from build123d import *

# Parameters (mm, degrees)
SKETCH1_R           = 1.1
SKETCH1_R_2         = 1.55
BOSS_EXTRUDE1_DEPTH = 2
SKETCH2_R           = 1.55
SKETCH2_R_2         = 1.1
BOSS_EXTRUDE2_DEPTH = 2.5
BOSS_EXTRUDE3_START = -3
SKETCH3_W           = 15.5
SKETCH3_H           = 3.5
BOSS_EXTRUDE3_DEPTH = 3
SKETCH4_R           = 1.5
CUT_EXTRUDE1_DEPTH  = 5
CUT_EXTRUDE2_DEPTH  = 65.325422657
CUT_EXTRUDE3_DEPTH  = 106.250938238
CHAMFER1_SIZE       = 2.5


with BuildPart() as part:
    # Sketch1 → Boss-Extrude1 (new body)
    with BuildSketch(Plane(origin=(0, 0, 0), x_dir=(1, 0, 0), z_dir=(0, 1, 0))):
        with BuildLine():
            Line((-48, -42.4), (-43, -42.4))
            Line((-43, -42.4), (-35.267949192, -37.935898385))
            ThreePointArc((-35.267949192, -37.935898385), (-34.303225373, -37.536296695), (-33.267949192, -37.4))
            Line((-33.267949192, -37.4), (33.267949192, -37.4))
            ThreePointArc((33.267949192, -37.4), (34.303225373, -37.536296695), (35.267949192, -37.935898385))
            Line((35.267949192, -37.935898385), (43, -42.4))
            Line((43, -42.4), (48, -42.4))
            Line((48, -42.4), (48, 42.4))
            Line((48, 42.4), (43, 42.4))
            Line((43, 42.4), (35.267949192, 37.935898385))
            ThreePointArc((35.267949192, 37.935898385), (34.303225373, 37.536296695), (33.267949192, 37.4))
            Line((33.267949192, 37.4), (-33.267949192, 37.4))
            ThreePointArc((-33.267949192, 37.4), (-34.303225373, 37.536296695), (-35.267949192, 37.935898385))
            Line((-35.267949192, 37.935898385), (-43, 42.4))
            Line((-43, 42.4), (-48, 42.4))
            Line((-48, 42.4), (-48, -42.4))
        make_face()
        with Locations(Location((-13.5, -33.275, 0), (0, 0, 270))):
            Circle(SKETCH1_R, mode=Mode.SUBTRACT)
        with Locations(Location((-7.5, -33.275, 0), (0, 0, 270))):
            Circle(SKETCH1_R, mode=Mode.SUBTRACT)
        with Locations(Location((7.5, -33.275, 0), (0, 0, 270))):
            Circle(SKETCH1_R, mode=Mode.SUBTRACT)
        with Locations(Location((13.5, -33.275, 0), (0, 0, 270))):
            Circle(SKETCH1_R, mode=Mode.SUBTRACT)
        with Locations(Location((-13.5, 33.275, 0), (0, 0, 270))):
            Circle(SKETCH1_R, mode=Mode.SUBTRACT)
        with Locations(Location((-7.5, 33.275, 0), (0, 0, 270))):
            Circle(SKETCH1_R, mode=Mode.SUBTRACT)
        with Locations(Location((7.5, 33.275, 0), (0, 0, 270))):
            Circle(SKETCH1_R, mode=Mode.SUBTRACT)
        with Locations(Location((13.5, 33.275, 0), (0, 0, 270))):
            Circle(SKETCH1_R, mode=Mode.SUBTRACT)
        with Locations(Location((-42, 36.5, 0), (0, 0, 270))):
            Circle(SKETCH1_R_2, mode=Mode.SUBTRACT)
        with Locations(Location((42, 36.5, 0), (0, 0, 270))):
            Circle(SKETCH1_R_2, mode=Mode.SUBTRACT)
        with Locations(Location((42, -36.5, 0), (0, 0, 270))):
            Circle(SKETCH1_R_2, mode=Mode.SUBTRACT)
        with Locations(Location((-42, -36.5, 0), (0, 0, 270))):
            Circle(SKETCH1_R_2, mode=Mode.SUBTRACT)
        with BuildLine():
            Line((-37, 25.25), (-37, 9.75))
            ThreePointArc((-37, 9.75), (-41, 5.75), (-45, 9.75))
            Line((-45, 9.75), (-45, 25.25))
            ThreePointArc((-45, 25.25), (-41, 29.25), (-37, 25.25))
        make_face(mode=Mode.SUBTRACT)
        with BuildLine():
            Line((-37, -9.75), (-37, -25.25))
            ThreePointArc((-37, -25.25), (-41, -29.25), (-45, -25.25))
            Line((-45, -25.25), (-45, -9.75))
            ThreePointArc((-45, -9.75), (-41, -5.75), (-37, -9.75))
        make_face(mode=Mode.SUBTRACT)
        with BuildLine():
            Line((45, 25.25), (45, 9.75))
            ThreePointArc((45, 9.75), (41, 5.75), (37, 9.75))
            Line((37, 9.75), (37, 25.25))
            ThreePointArc((37, 25.25), (41, 29.25), (45, 25.25))
        make_face(mode=Mode.SUBTRACT)
        with BuildLine():
            Line((45, -9.75), (45, -25.25))
            ThreePointArc((45, -25.25), (41, -29.25), (37, -25.25))
            Line((37, -25.25), (37, -9.75))
            ThreePointArc((37, -9.75), (41, -5.75), (45, -9.75))
        make_face(mode=Mode.SUBTRACT)
    extrude(amount=BOSS_EXTRUDE1_DEPTH)

    # Sketch2 → Boss-Extrude2 (add)
    with BuildSketch(Plane(origin=(0, 2, 0), x_dir=(1, 0, 0), z_dir=(0, 1, 0))):
        with BuildLine():
            Line((48, -42.4), (48, 42.4))
            Line((48, 42.4), (43, 42.4))
            Line((43, 42.4), (35.267949192, 37.935898385))
            ThreePointArc((35.267949192, 37.935898385), (34.303225373, 37.536296695), (33.267949192, 37.4))
            Line((33.267949192, 37.4), (-33.267949192, 37.4))
            ThreePointArc((-33.267949192, 37.4), (-34.303225373, 37.536296695), (-35.267949192, 37.935898385))
            Line((-35.267949192, 37.935898385), (-43, 42.4))
            Line((-43, 42.4), (-48, 42.4))
            Line((-48, 42.4), (-48, -42.4))
            Line((-48, -42.4), (-43, -42.4))
            Line((-43, -42.4), (-35.267949192, -37.935898385))
            ThreePointArc((-35.267949192, -37.935898385), (-34.303225373, -37.536296695), (-33.267949192, -37.4))
            Line((-33.267949192, -37.4), (33.267949192, -37.4))
            ThreePointArc((33.267949192, -37.4), (34.303225373, -37.536296695), (35.267949192, -37.935898385))
            Line((35.267949192, -37.935898385), (43, -42.4))
            Line((43, -42.4), (48, -42.4))
        make_face()
        with Locations((-42, -36.5)):
            Circle(SKETCH2_R, mode=Mode.SUBTRACT)
        with Locations((-13.5, -33.275)):
            Circle(SKETCH2_R_2, mode=Mode.SUBTRACT)
        with Locations((-7.5, -33.275)):
            Circle(SKETCH2_R_2, mode=Mode.SUBTRACT)
        with Locations((7.5, -33.275)):
            Circle(SKETCH2_R_2, mode=Mode.SUBTRACT)
        with Locations((13.5, -33.275)):
            Circle(SKETCH2_R_2, mode=Mode.SUBTRACT)
        with Locations((42, -36.5)):
            Circle(SKETCH2_R, mode=Mode.SUBTRACT)
        with Locations((-42, 36.5)):
            Circle(SKETCH2_R, mode=Mode.SUBTRACT)
        with Locations((-13.5, 33.275)):
            Circle(SKETCH2_R_2, mode=Mode.SUBTRACT)
        with Locations((-7.5, 33.275)):
            Circle(SKETCH2_R_2, mode=Mode.SUBTRACT)
        with BuildLine():
            Line((45, 9.75), (45, -9.75))
            Line((45, -9.75), (45, -25.25))
            ThreePointArc((45, -25.25), (43.828427125, -28.078427125), (41, -29.25))
            Line((41, -29.25), (-41, -29.25))
            ThreePointArc((-41, -29.25), (-43.828427125, -28.078427125), (-45, -25.25))
            Line((-45, -25.25), (-45, -9.75))
            Line((-45, -9.75), (-45, 9.75))
            Line((-45, 9.75), (-45, 25.25))
            ThreePointArc((-45, 25.25), (-43.828427125, 28.078427125), (-41, 29.25))
            Line((-41, 29.25), (41, 29.25))
            ThreePointArc((41, 29.25), (43.828427125, 28.078427125), (45, 25.25))
            Line((45, 25.25), (45, 9.75))
        make_face(mode=Mode.SUBTRACT)
        with Locations((7.5, 33.275)):
            Circle(SKETCH2_R_2, mode=Mode.SUBTRACT)
        with Locations((13.5, 33.275)):
            Circle(SKETCH2_R_2, mode=Mode.SUBTRACT)
        with Locations((42, 36.5)):
            Circle(SKETCH2_R, mode=Mode.SUBTRACT)
    extrude(amount=BOSS_EXTRUDE2_DEPTH)

    # Sketch3 → Boss-Extrude3 (add)
    with BuildSketch(Plane(origin=(48, 0, 0), x_dir=(0, 0, -1), z_dir=(1, 0, 0)).offset(BOSS_EXTRUDE3_START)):
        with Locations((-17.5, 6.25)):
            Rectangle(SKETCH3_W, SKETCH3_H)
        with Locations((17.5, 6.25)):
            Rectangle(SKETCH3_W, SKETCH3_H)
    boss_extrude3 = extrude(amount=BOSS_EXTRUDE3_DEPTH)

    # Sketch4 → Cut-Extrude1 (cut)
    with BuildSketch(Plane(origin=(48, 0, 0), x_dir=(0, 0, -1), z_dir=(1, 0, 0))):
        with Locations((-17.5, 4)):
            Circle(SKETCH4_R)
        with Locations((17.5, 4)):
            Circle(SKETCH4_R)
    cut_extrude1 = extrude(amount=-CUT_EXTRUDE1_DEPTH, mode=Mode.SUBTRACT)

    # Mirror1: Boss-Extrude3, Cut-Extrude1 across plane
    add(boss_extrude3.mirror(Plane(origin=(0, 0, 0), x_dir=(0, 0, 1), z_dir=(1, 0, 0))))
    add(cut_extrude1.mirror(Plane(origin=(0, 0, 0), x_dir=(0, 0, 1), z_dir=(1, 0, 0))), mode=Mode.SUBTRACT)

    # Sketch5 → Cut-Extrude2 (cut, through all)
    with BuildSketch(Plane(origin=(0, 2, 0), x_dir=(1, 0, 0), z_dir=(0, 1, 0))):
        with BuildLine():
            Line((-24.387725676, -18.900172978), (-7.47454864, -2.130327951))
            ThreePointArc((-7.47454864, -2.130327951), (-6.586822965, 0), (-7.47454864, 2.130327951))
            Line((-7.47454864, 2.130327951), (-24.387725676, 18.900172978))
            ThreePointArc((-24.387725676, 18.900172978), (-27.653944762, 19.539034707), (-29.5, 16.769845027))
            Line((-29.5, 16.769845027), (-29.5, -16.769845027))
            ThreePointArc((-29.5, -16.769845027), (-27.653944762, -19.539034707), (-24.387725676, -18.900172978))
        make_face()
        with BuildLine():
            Line((18.999810334, 24.119672049), (2.112274324, 7.375250751))
            ThreePointArc((2.112274324, 7.375250751), (0, 6.505578702), (-2.112274324, 7.375250751))
            Line((-2.112274324, 7.375250751), (-18.999810334, 24.119672049))
            ThreePointArc((-18.999810334, 24.119672049), (-19.661610977, 27.392150635), (-16.88753601, 29.25))
            Line((-16.88753601, 29.25), (16.88753601, 29.25))
            ThreePointArc((16.88753601, 29.25), (19.661610977, 27.392150635), (18.999810334, 24.119672049))
        make_face()
        with BuildLine():
            Line((-18.999810334, -24.119672049), (-2.112274324, -7.375250751))
            ThreePointArc((-2.112274324, -7.375250751), (0, -6.505578702), (2.112274324, -7.375250751))
            Line((2.112274324, -7.375250751), (18.999810334, -24.119672049))
            ThreePointArc((18.999810334, -24.119672049), (19.661610977, -27.392150635), (16.88753601, -29.25))
            Line((16.88753601, -29.25), (-16.88753601, -29.25))
            ThreePointArc((-16.88753601, -29.25), (-19.661610977, -27.392150635), (-18.999810334, -24.119672049))
        make_face()
        with BuildLine():
            Line((7.47454864, 2.130327951), (24.387725676, 18.900172978))
            ThreePointArc((24.387725676, 18.900172978), (27.653944762, 19.539034707), (29.5, 16.769845027))
            Line((29.5, 16.769845027), (29.5, -16.769845027))
            ThreePointArc((29.5, -16.769845027), (27.653944762, -19.539034707), (24.387725676, -18.900172978))
            Line((24.387725676, -18.900172978), (7.47454864, -2.130327951))
            ThreePointArc((7.47454864, -2.130327951), (6.586822965, 0), (7.47454864, 2.130327951))
        make_face()
    extrude(amount=-CUT_EXTRUDE2_DEPTH, mode=Mode.SUBTRACT)

    # Sketch6 → Cut-Extrude3 (cut, through all)
    with BuildSketch(Plane.ZY.offset(48)):
        Polygon((-25.25, 4.5), (-21.75, 8), (-25.25, 8), align=None)
        Polygon((-9.75, 4.5), (-13.25, 8), (-9.75, 8), align=None)
        Polygon((9.75, 4.5), (9.75, 8), (13.25, 8), align=None)
        Polygon((25.25, 4.5), (25.25, 8), (21.75, 8), align=None)
    extrude(amount=-CUT_EXTRUDE3_DEPTH, mode=Mode.SUBTRACT)

    # Chamfer1
    chamfer1_edges = [part.edges().sort_by_distance(p)[0] for p in [
        (45, 2, 0),
        (-45, 2, 0),
    ]]
    chamfer(chamfer1_edges, length=CHAMFER1_SIZE - 0.0001)  # a hair under: the kernel refuses the full size


solid = part.part
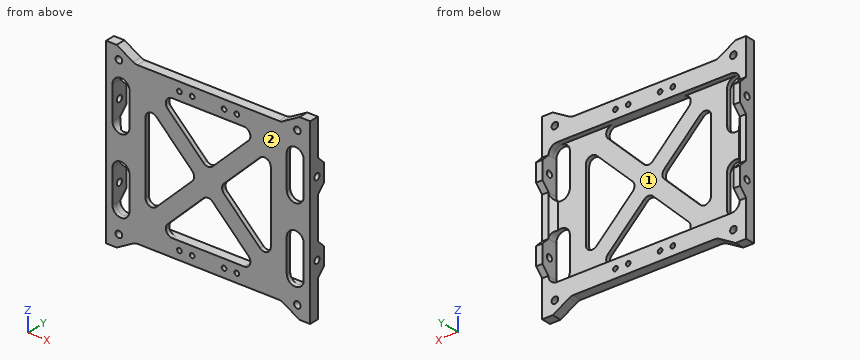
The model under review builds one solid part; all positions refer to its coordinate system, in mm. Face numbers are marked on the shaded views. A direction names the side the tool comes from. Coordinates: 2 decimals unless noted, no trailing zeros. Write each loop counter-clockwise with the first axis right and the second up, starting at its lowest first coordinate (ties: lowest second). Pieces come first, ordered by that corner, then holes. Notation, with made-up numbers: (41, -40) - (55, -40) arc R26 ccw to (55, -13) - close; hole circle Ø2 at (-7.5, 37). An arc over 180 degrees is marked (long way). Answer as a JSON object with one key per item and string values. Group by question number.
1. Add section A-A (z = 0). Give the number of separate pieces and of enclosed holes in the cut face, plus the area to 3 significant figures.
2. Clearance check with flat-ended pins moving along their axes: pin 1 Ø1.8 at (x, z) = (7.5, -33.275) entering from -Y; pin 2 Ø4 at (x, z) = (42, 36.5) entering from +Y; pin 3 Ø3 at (x, y) = (-1, 2) entering from -Z; pin 4 Ø1.3 at (x, y) = (-1, 2.5) entering from +Z. State where each tip first meets the part, or that it passes through.
3. To check wall thickness, follow probe 1 along X at (y, z) = (3, -36.5); probe 2 along Z at (x, y) = (-46.9, 4); probe 3 along Z at (x, y) = (7.5, 2.15) (3 decimals). State the ranges of each line that lie inside material, in increasing order.
4. Add section C-C (x = 5). Give the boundary of the cut face in (y, z).
5. Machinability: for the marked faces 1 and 2, which of the approach directions +Z, -Z, +X, -X, +Y, -Y give a long, thin tool a straight path to every point of the face, cutting with its end or side? Answer none if there is none.
6. Add section B-B (z = 14.5). Give the boundary of the cut face in (x, y), plus the area to 3 significant figures.
Findings:
{
 "1": {"separate pieces": "3", "enclosed holes": "0", "area": "122 mm²"},
 "2": {"pin 1": "through", "pin 2": "y = 4.5", "pin 3": "z = -37.4", "pin 4": "z = 37.4"},
 "3": {"probe 1": "-48 to -43.55, -40.45 to 40.45, 43.55 to 48", "probe 2": "-42.4 to -19, -16 to 16, 19 to 42.4", "probe 3": "-37.4 to -34.375, -32.175 to -29.25, 29.25 to 32.175, 34.375 to 37.4"},
 "4": {"outline": "(0, -37.4) - (4.5, -37.4) - (4.5, -29.25) - (0, -29.25) - close; (0, -10.24) - (2, -10.24) - (2, 10.24) - (0, 10.24) - close; (0, 29.25) - (4.5, 29.25) - (4.5, 37.4) - (0, 37.4) - close"},
 "5": {"face 1": "+Y", "face 2": "+Z, -Z, +X, -X, -Y"},
 "6": {"outline": "(-48, 0) - (-45, 0) - (-45, 8) - (-48, 8) - close; (-37, 0) - (-29.5, 0) - (-29.5, 2) - (-37, 2) - close; (-19.95, 0) - (-9.3, 0) - (-9.3, 2) - (-19.95, 2) - close; (9.3, 0) - (19.95, 0) - (19.95, 2) - (9.3, 2) - close; (29.5, 0) - (37, 0) - (37, 2) - (29.5, 2) - close; (45, 0) - (48, 0) - (48, 8) - (45, 8) - close", "area": "121 mm²"}
}
